Geometry: final body of the model. Coordinates: model frame, mm. A direction names the side the tool comes from. Give positions to 0.01 mm unless a question says otherwise; leave off trailing zeros. Write each loop counter-clockwise with the first axis right and the second up, starting at its lowest first coordinate (ties: lowest second). Pieces come first, ordered by that corner, then holes. Notation, with made-up numbers: (48, 52.5) -> (67, 52.5) arc R23 ccw to (67, 64.5) -> close; hole circle Ø9 at (14.25, -5.5). An arc over 180 degrees is marked (long way). Answer in a Markdown table with one row per item. Add a question column.
Item 1: Material intervals for probe 1 along X at (y, z) = (-61.5, 0.55); probe 2 along Y at (x, z) = (-5, 0.4); probe 3 along Y at (x, z) = (-33.25, 1.15), sorted ascending. Write a range as from..to.
Item 2: Access query for faces 1 (the cylindrical face through (-20.675, 49.536, -0.028)), 2 (the flat face through (-33, 35, 0)). Directions: +Z, -Z, +X, -X, +Y, -Y. A direction counts if a zero-diameter tool reaches every point of the face in a straight line with its end or side. Return the directions, or none.
Item 3: Section query C-C on z = -0.15. State how many separate pieces and enclosed holes the cut face has, plus the area to 3 significant figures.
Item 4: Section query B-B on x = 11. Output: boundary loops of the cut face in (y, z), plus the area to 3 significant figures.
Item 5: Draft query along X for faces 3 (the flat face through (-40, -25, 0)), 4 (the flat face through (40, 2, 0)), 5 (the flat face through (-31, 25, 0)), 6 (the cylindrical face through (11.325, 49.536, -0.028)). Return one class per face: +X half, -X half, draft (parallel to the pull), parting line (faces both ways), or undercut.
Item 6: Section query A-A on y = 1. Output: boundary loops of the cut face in (x, z).
Item 7: First-contact query: P1, Ø1.8, axis at x = 11, y = 19, coming from the -Z side. Flat tip, straight axial feed; report the tip coordinate or a pass-through.
Item 8: Section query D-D on x = 33.25. Output: boundary loops of the cut face in (y, z).
Autodesk Inventor part; units mm, degrees
ref_plane "YZ Plane" through (0, 0, 0) normal (1, 0, 0) x (0, 1, 0)
ref_plane "XZ Plane" through (0, 0, 0) normal (0, 1, 0) x (-1, 0, 0)
ref_plane "XY Plane" through (0, 0, 0) normal (0, 0, 1) x (1, 0, 0)
sketch "Sketch1" plane through (0, 0, 0) normal (0, 0, 1) x (-1, 0, 0)
  line L0 (-38, 74) -> (38, 74)
  line L1 (40, 72) -> (40, -74)
  line L2 (40, -74) -> (-40, -74)
  line L3 (-40, -74) -> (-40, 72)
  circle A0 centre (-33.25, 61.5) radius 1.65
  circle A1 centre (33.25, 61.5) radius 1.65
  circle A2 centre (33.25, -57.5) radius 1.65
  circle A3 centre (-33.25, -57.5) radius 1.65
  line L4 (-33.25, 61.5) -> (33.25, 61.5) construction
  line L5 (33.25, 61.5) -> (33.25, -57.5) construction
  circle A4 centre (5, 35) radius 20
  circle A5 centre (5, -35) radius 20
  line L6 (5, 35) -> (5, -35) construction
  line L7 (-11, -51) -> (21, -51) construction
  line L8 (21, -51) -> (21, -19) construction
  line L9 (-11, 51) -> (21, 51) construction
  line L10 (21, 51) -> (21, 19) construction
  circle A6 centre (-11, 51) radius 1.5
  circle A7 centre (21, 51) radius 1.5
  circle A8 centre (21, 19) radius 1.5
  circle A9 centre (-11, 19) radius 1.5
  circle A10 centre (21, -19) radius 1.5
  circle A11 centre (21, -51) radius 1.5
  circle A12 centre (-11, -51) radius 1.5
  circle A13 centre (-11, -19) radius 1.5
  arc A14 (-38, 74) -> (-40, 72) centre (-38, 72) ccw
  arc A15 (40, 72) -> (38, 74) centre (38, 72) ccw
  point P0 (0, 0)
  point P1 (-40, 74)
  point P2 (40, 74)
  point P3 (0, 74)
  point P4 (-40, 0)
  point P5 (0, 61.5)
  point P6 (5, 0)
  point P7 (21, 35)
  point P8 (5, 51)
  point P9 (5, -51)
  point P10 (21, -35)
  dimension "d15" = 2
  dimension "d0" = 80
  dimension "d1" = 148
  dimension "d2" = 3.3
  dimension "d3" = 119
  dimension "d4" = 66.5
  dimension "d20" = 40
  dimension "d21" = 40
  dimension "d22" = 70
  dimension "d23" = 32
  dimension "d24" = 3
  dimension "d26" = 5
  dimension "d28" = 2
  dimension "d29" = 16.5
  dimension "d30" = 74
extrude "soporte circuito KAEN" add sketch "Sketch1" along normal mid plane 4
sketch "Sketch2" plane through (0, 0, 2) normal (0, 0, 1) x (-1, 0, 0)
  line L0 (-20, -1) -> (20, -1) construction
  line L1 (40, -74) -> (40, 72) construction
  line L2 (-40, -74) -> (40, -74)
  point P0 (0, 0)
  point P1 (36.5, 73)
  point P2 (0, -1)
  point P3 (36.5, -74)
  point P4 (-36.5, -74)
  point P5 (34.5, -75)
  point P6 (40, 72)
  dimension "d11" = 40
  dimension "d25" = 73
hole "M5" at (20, 1, 2) at (-20, 1, 2) direction (0, 0, -1) diameter 4.134 end through all
sketch "Sketch3" plane through (0, 0, 2) normal (0, 0, 1) x (1, 0, 0)
  line L0 (-41, 35) -> (-22, 35)
  line L1 (-22, 35) -> (-22, 25)
  line L2 (-22, 25) -> (-41, 25)
  line L3 (-41, 25) -> (-41, 35)
  circle A0 centre (-5, 35) radius 20
  point P0 (0, 0)
  point P1 (-31.5, 35)
  point P2 (-22.3205, 25)
  point P3 (-25, 35)
  dimension "d31" = 10
  dimension "d32" = 19
  dimension "d33" = 17
extrude "Extrusion2" cut sketch "Sketch3" against normal through all contours L0 A0 L2 L3
fillet "Fillet2" radius 2 4 edges at (-40, 35, 0) (-40, 25, 0) (-25, 35, 0) (-22.3205, 25, 0)
properties part number "Placa soporte TIC DC" material "Polycarbonate, Smoke"
Findings below:
| question | item | result |
|---|---|---|
| 1 | probe 1 | x = -40..-34.9, -31.6..31.6, 34.9..40 |
| 1 | probe 2 | y = -74..-55, -15..15, 55..74 |
| 1 | probe 3 | y = -74..-63.15, -59.85..25, 35..55.85, 59.15..74 |
| 2 | face 1 | +Z, -Z |
| 2 | face 2 | +Z, -Z, -X |
| 3 | separate pieces | 1 |
| 3 | enclosed holes | 15 |
| 3 | area | 9,050 mm^2 |
| 4 | outline | (-74, -2) -> (-52.5, -2) -> (-52.5, 2) -> (-74, 2) -> close; (-49.5, -2) -> (-47, -2) -> (-47, 2) -> (-49.5, 2) -> close; (-23, -2) -> (-20.5, -2) -> (-20.5, 2) -> (-23, 2) -> close; (-17.5, -2) -> (17.5, -2) -> (17.5, 2) -> (-17.5, 2) -> close; (20.5, -2) -> (23, -2) -> (23, 2) -> (20.5, 2) -> close; (47, -2) -> (49.5, -2) -> (49.5, 2) -> (47, 2) -> close; (52.5, -2) -> (74, -2) -> (74, 2) -> (52.5, 2) -> close |
| 4 | area | 352 mm^2 |
| 5 | face 3 | -X half |
| 5 | face 4 | +X half |
| 5 | face 5 | draft |
| 5 | face 6 | undercut |
| 6 | outline | (-40, -2) -> (-22.07, -2) -> (-22.07, 2) -> (-40, 2) -> close; (-17.93, -2) -> (17.93, -2) -> (17.93, 2) -> (-17.93, 2) -> close; (22.07, -2) -> (40, -2) -> (40, 2) -> (22.07, 2) -> close |
| 7 | P1 | passes through |
| 8 | outline | (-74, -2) -> (-63.15, -2) -> (-63.15, 2) -> (-74, 2) -> close; (-59.85, -2) -> (55.85, -2) -> (55.85, 2) -> (-59.85, 2) -> close; (59.15, -2) -> (74, -2) -> (74, 2) -> (59.15, 2) -> close |
